Build history of the part. All positions in model axes, mm. Round coordinates to 2 decimals unless told otherwise and drop trailing zeros. Write each loop counter-clockwise with the first axis right and the second up, starting at its lowest first coordinate (ties: lowest second). Pieces come first, ordered by that corner, then holes.
Item 1: Band-saw the part on B-B, the plane z = 0. Write the cut outline in (x, y), then the cut area to 3 significant figures.
Item 2: Wall check: probe 1 along X at (y, z) = (0.4, 0); probe 2 along Z at (x, y) = (3.5, 0.15); probe 3 along Z at (x, y) = (-7, 0.5). Give the ranges that are in metal, low to high.
Item 3: Mould opens along Z. For faces 1 (the conical face through (3.05, 0.65, 9.68)), 2 (the flat face through (-12.3, 0.5, -15)), 3 (the flat face through (-12.7, 0.5, 15)) say: +Z half, -Z half, draft (parallel to the pull), parting line (faces both ways), or undercut.
Item 4: Drop a flat-ended pin along its axis: pin 1 Ø3 at (x, z) = (-3.5, -10.5) entering from +Y. Give the stop position or say it passes through.
Item 5: Band-saw the part on A-A, the plane y = 0.35. Write the cut outline in (x, z), then the cut area to 3 significant figures.
```python
from build123d import *

# Parameters (mm, degrees)
SKETCH1_R           = 10
BOSS_EXTRUDE1_DEPTH = 1
CHAMFER1_SIZE       = 3
CHAMFER1_SIZE2      = 0.368353683


with BuildPart() as part:
    # Sketch1 → Boss-Extrude1 (new body)
    with BuildSketch(Plane(origin=(0, 0, 0), x_dir=(1, 0, 0), z_dir=(0, 1, 0))):
        with BuildLine():
            Line((0, 15), (-25, 15))
            ThreePointArc((-25, 15), (-28.535533906, 13.535533906), (-30, 10))
            Line((-30, 10), (-30, -10))
            ThreePointArc((-30, -10), (-28.535533906, -13.535533906), (-25, -15))
            Line((-25, -15), (0, -15))
            ThreePointArc((0, -15), (15, 0), (0, 15))
        make_face()
        with Locations(Location((0, 0, 0), (0, 0, 270))):
            Circle(SKETCH1_R, mode=Mode.SUBTRACT)
    extrude(amount=BOSS_EXTRUDE1_DEPTH)

    # Chamfer1
    chamfer1_edges = [part.edges().sort_by_distance(p)[0] for p in [
        (0, 1, -10),
    ]]
    chamfer1_side = [part.faces().sort_by_distance(p)[0] for p in [
        (-11.782026839, 1, 0),
    ]]
    chamfer(chamfer1_edges, length=CHAMFER1_SIZE, length2=CHAMFER1_SIZE2, reference=chamfer1_side[0])


solid = part.part
```
Results:
1. outline: (-30, 0) - (-10, 0) - (-10, 0.63) - (-13, 1) - (-30, 1) - close; (10, 0) - (15, 0) - (15, 1) - (13, 1) - (10, 0.63) - close
1. area: 23.9 mm2
2. probe 1: x = -30 to -10, 10 to 15
2. probe 2: z = -14.59 to -9.37, 9.37 to 14.59
2. probe 3: z = -15 to -7.14, 7.14 to 15
3. face 1: undercut
3. face 2: -Z half
3. face 3: +Z half
4. pin 1: stops at y = 0.95
5. outline: (-30, -10) arc R5 ccw to (-25, -15) - (0, -15) arc R15 ccw to (0, 15) - (-25, 15) arc R5 ccw to (-30, 10) - close; hole circle Ø20 at (0, 0)
5. area: 929 mm2
